Source: three-view drawing plus pictorial views. Frame: mm from the lowest corner of the part. A direction names the side the tool comes from. Give positions to 0.01 mm unless a question says otherwise; leave off trailing zeros. Loops run counter-clockwise (first coordinate to the right, second up) from the corner with the lowest first, then second, coordinate; pieces in that order, holes last. Notation, with made-up numbers: (-36, -17.75) - (-28, -17.75) arc R8 ccw to (-28, -2.75) - close; hole circle Ø5 at (16, -5). An arc over 180 degrees is marked (long way). One line per item, written item: value.
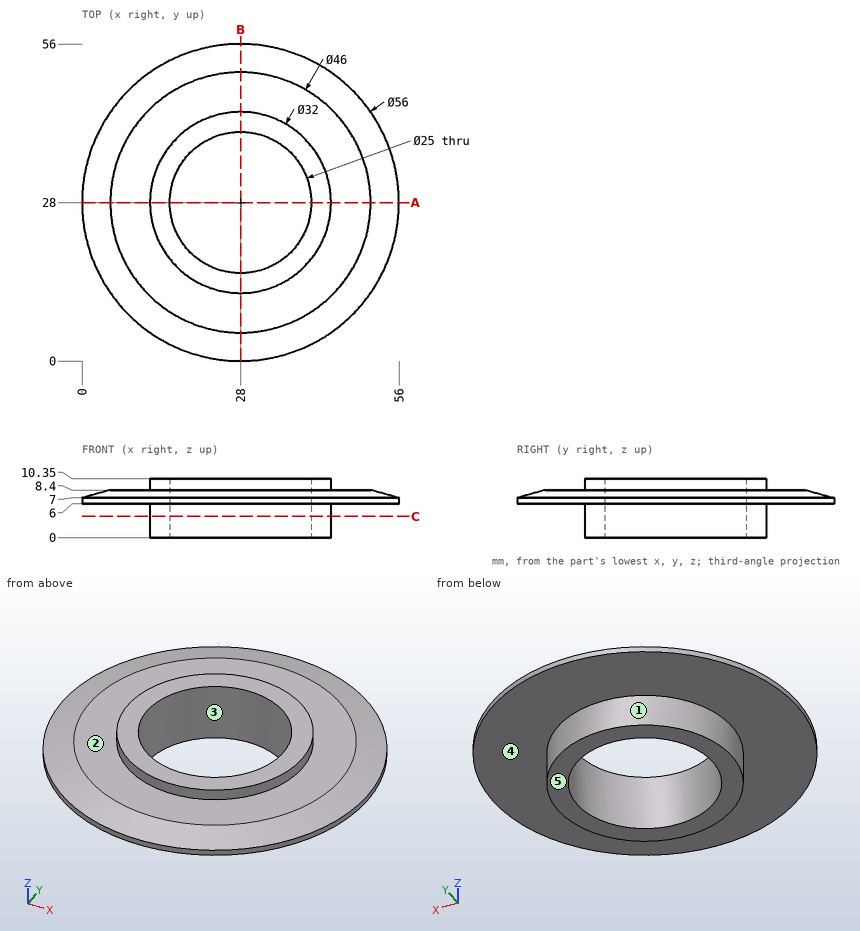
Item 1: Access query for the marked faces 4 and 5. Directions: +Z, -Z, +X, -X, +Y, -Y. A direction counts if a zero-diameter tool reaches every point of the face in a straight line with its end or side. Return the directions, or none.
Verdict:
face 4: -Z
face 5: -Z, +X, -X, +Y, -Y
Item 2: Section A-A, the plane y = 28. Output: boundary loops of the cut face in (x, z), and give its area (3 significant figures).
Verdict:
outline: (0, 6) - (12, 6) - (12, 0) - (15.5, 0) - (15.5, 10.35) - (12, 10.35) - (12, 8.4) - (5, 8.4) - (0, 7) - close; (40.5, 0) - (44, 0) - (44, 6) - (56, 6) - (56, 7) - (51, 8.4) - (44, 8.4) - (44, 10.35) - (40.5, 10.35) - close
area: 123 mm^2
Item 3: Pin query (flat end, axial travel): P1, Ø2, axis at x = 43.5, y = 41.5, coming from the +Z side; P2, Ø6, axis at y = 20.5, z = 2.5, coming from the -X side; P3, Ø3, axis at y = 49, z = 5, coming from the -X side; P4, Ø10, axis at x = 39.5, y = 14.5, coming from the -Z side. Return the tip coordinate at first contact, or that it passes through.
Verdict:
P1: stops at z = 8.4
P2: stops at x = 12.65
P3: stops at x = 8.28
P4: stops at z = 0
Item 4: Section C-C, the plane z = 3.75. Output: boundary loops of the cut face in (x, y).
Verdict:
outline: circle Ø32 at (28, 28); hole circle Ø25 at (28, 28)
Item 5: Draft query along X for the marked faces 1, 2 and 3. Return one class per face: pulls with the +X half, pulls with the -X half, needs draft (parallel to the pull), parting line crosses it, or undercut.
Verdict:
face 1: parting line crosses it
face 2: needs draft
face 3: undercut
Item 6: Material intervals for L1, parallel to Y at x = 28, z = 3.5; L2, parallel to Z at x = 30, y = 5.5; L3, parallel to Y at x = 25.5, z = 4.5, sorted ascending.
Verdict:
L1: y = 12 to 15.5, 40.5 to 44
L2: z = 6 to 8.4
L3: y = 12.2 to 15.75, 40.25 to 43.8
